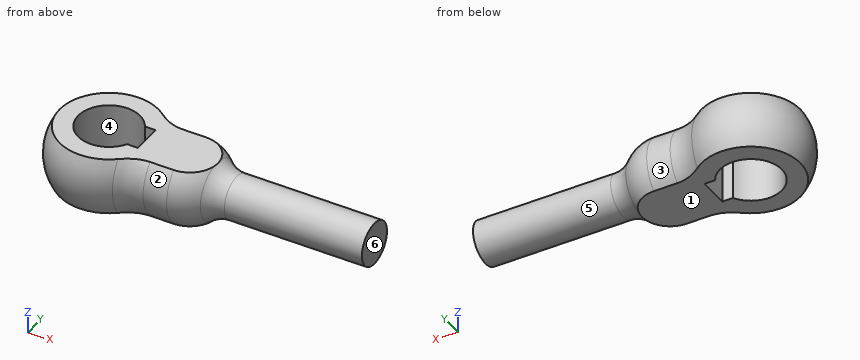
Autodesk Inventor part; units mm, degrees
ref_plane "YZ Plane" through (0, 0, 0) normal (1, 0, 0) x (0, 1, 0)
ref_plane "XZ Plane" through (0, 0, 0) normal (0, 1, 0) x (-1, 0, 0)
ref_plane "XY Plane" through (0, 0, 0) normal (0, 0, 1) x (1, 0, 0)
sketch "Эскиз1" plane through (0, 0, 0) normal (0, 0, 1) x (1, 0, 0)
  circle A0 centre (0, 0) radius 60
  circle A1 centre (0, 0) radius 32.5
  line L0 (28.2887, 16) -> (28.2887, -16)
  line L1 (28.2887, 16) -> (39.5, 16)
  line L2 (39.5, 16) -> (39.5, -16)
  line L3 (39.5, -16) -> (28.2887, -16)
  line L4 (-60, 0) -> (279.451, 0)
  line L5 (42.8486, 42) -> (42.8486, -42)
  line L6 (42.8486, 42) -> (85, 42)
  line L7 (85, 42) -> (85, -42)
  line L8 (85, -42) -> (42.8486, -42)
  line L9 (42.8486, -42) -> (42.8486, 42)
  circle A2 centre (60.2993, 92) radius 50
  line L10 (0, 0) -> (60.2993, 92)
  circle A3 centre (85, 0) radius 42
  line L11 (85, 22.5) -> (278.9533, 22.5)
  line L12 (278.9533, 22.5) -> (278.9533, -22.5)
  line L13 (278.9533, -22.5) -> (85, -22.5)
  line L14 (85, -22.5) -> (85, 22.5)
  circle A4 centre (134.2722, 52.5) radius 30
  line L15 (85, 0) -> (134.2722, 52.5)
  point P0 (-32.5, 0)
  point P1 (278.9533, 0)
  point P2 (278.9533, 0)
  point P3 (134.2722, 22.5)
  point P4 (113.7421, 30.625)
  point P5 (60.2993, 42)
  point P6 (32.8905, 50.1818)
  dimension "d17" = 84
  dimension "d0" = 120
  dimension "d1" = 65
  dimension "d2" = 32
  dimension "d3" = 72
  dimension "d4" = 84
  dimension "d7" = 100
  dimension "d8" = 92
  dimension "d10" = 110
  dimension "d11" = 85
  dimension "d12" = 0
  dimension "d13" = 45
  dimension "d14" = 60
  dimension "d15" = 52.5
  dimension "d16" = 72
  dimension "d18" = 0
revolve "Вращение1" add sketch "Эскиз1" angle 360 about axis through (-60, 0, 0) along (1, 0, 0) picked at (45.8038, 26.0598) picked at (54.3043, 5.6582) picked at (76.4143, 10.6672) picked at (29.0608, 8.9784) contours A0 L10 A1 L4 | A2 L6 A0 | A0 L5 L4 L2 L1 A1 L10 | A1 L10 L4 | L5 A0 A3 L4 | L6 A3 A0 | A1 L0 L4 L10 | L4 A3 A0 | A0 A3 L7 L4 | L4 A1 L1 L2 | A3 L15 L11 L7 | A1 L4 L0 | L15 L11 A3 L4 | L7 L11 L15 | A3 L11 L12 L4 | A4 L11 A3 | A3 L11 L15
sketch "Эскиз2" plane through (0, 0, 0) normal (0, 1, 0) x (-1, 0, 0)
  line L0 (105.3756, -30) -> (-295.1428, -30)
  line L1 (-295.1428, -30) -> (-295.1428, 30)
  line L2 (-295.1428, 30) -> (105.3756, 30)
  line L3 (105.3756, 30) -> (105.3756, -30)
  point P0 (0, 0)
  point P1 (105.3756, 0)
  point P2 (0, 0)
  dimension "d20" = 0
  dimension "d21" = 60
extrude "Выдавливание1" cut sketch "Эскиз2" along normal mid plane 200 keep common part
sketch "Эскиз3" plane through (60.2993, -29.3939, 30) normal (0, 0, 1) x (1, 0, 0)
  circle A0 centre (-60.2993, 29.3939) radius 32.5
  line L0 (-32.0106, 13.3939) -> (-32.0106, 45.3939)
  line L1 (-32.0106, 45.3939) -> (-20.7993, 45.3939)
  line L2 (-20.7993, 45.3939) -> (-20.7993, 13.3939)
  line L3 (-20.7993, 13.3939) -> (-32.0106, 13.3939)
  line L4 (-32.0106, 13.3939) -> (-32.0106, 45.3939)
  point P0 (-92.7993, 29.3939)
  point P1 (-32.0106, 13.3939)
  dimension "d24" = 65
  dimension "d25" = 32
  dimension "d26" = 72
extrude "Выдавливание2" cut sketch "Эскиз3" against normal blind 100
properties part number "1_3"
Input: part model. Units: mm. Frame: model coordinates. Face numbers are marked on the shaded views. A direction names the side the tool comes from. Coordinates: 2 decimals unless noted, no trailing zeros. Write each loop counter-clockwise with the first axis right and the second up, starting at its lowest first coordinate (ties: lowest second). Pieces come first, ordered by that corner, then holes. Notation, with made-up numbers: M -13.75,-14.75 L 30.25,-14.75 A20 ccw 30.25,1.25 Z; hole C 13.5,-3.75 d2. An arc over 180 degrees is marked long. Answer as a JSON object with one key per item and string values. Group by question number.
(1) Ray query, line 1 along Y through (x, z) = (11, -17.5); line 2 along X through (y, z) = (0.5, -17); line 3 along X through (y, z) = (-10.5, 19.5). Return the intervals inside material, ascending. Write a range as [from, to].
(2) Mould query, pull axis X, two halves, no side actions, for the marked faces 4, 5 and 6. Classes: pulls with the +X half, pulls with the -X half, needs draft (parallel to the pull), parting line crosses it, or undercut.
(3) Contact query for flat-ended pins moving along their axis: P1, Ø2, axis at x = 89.5, z = 0, coming from the -Y side; P2, Ø12, axis at x = 231.5, z = 6, coming from the -Y side; P3, Ø5.5, axis at x = 36, z = -7.5, coming from the +Y side. Output: stop coordinate, or through.
(4) Set-up query: the marked faces 1, 2 and 3. Return all of +Z, -Z, +X, -X, +Y, -Y with unobstructed straight access to the full face (end or side cutting, diameter ignored); none if empty.
(5) Section C-C on z = 0. Output: boundary loops of the cut face in (x, y) (3 decimals), plus the area to 3 significant figures.
(6) Section B-B on y = 0. Output: boundary loops of the cut face in (x, z), plus the area to 3 significant figures.
(7) Section D-D on x = 172.5. Output: boundary loops of the cut face in (y, z).
(8) Section A-A on x = 0. Output: boundary loops of the cut face in (y, z), plus the area to 3 significant figures.
Result set:
{
 "1": {"line 1": "y = [-56.33, -30.58], [30.58, 56.33]", "line 2": "x = [-57.54, -32.5], [39.5, 278.95]", "line 3": "x = [-55.76, -30.76], [39.5, 278.95]"},
 "2": {"face 4": "undercut", "face 5": "needs draft", "face 6": "pulls with the +X half"},
 "3": {"P1": "stops at y = -41.85", "P2": "stops at y = -22.5", "P3": "stops at y = 49.43"},
 "4": {"face 1": "-Z, +X, -X, +Y, -Y", "face 2": "+X, -Y", "face 3": "+X, +Y"},
 "5": {"outline": "M 32.891,-50.182 A50 cw 60.299,-42 L 85,-42 A42 ccw 113.742,-30.625 A30 cw 134.272,-22.5 L 278.953,-22.5 L 278.953,22.5 L 134.272,22.5 A30 cw 113.742,30.625 A42 ccw 85,42 L 60.299,42 A50 cw 32.891,50.182 A60 ccw long Z; hole M 28.289,-16 L 39.5,-16 L 39.5,16 L 28.289,16 A32.5 ccw long Z", "area": "20,100 mm2"},
 "6": {"outline": "M -51.96,-30 L -32.5,-30 L -32.5,30 L -51.96,30 A60 ccw Z; M 39.5,-30 L 114.43,-30 A30 cw 134.27,-22.5 L 278.95,-22.5 L 278.95,22.5 L 134.27,22.5 A30 cw 114.43,30 L 39.5,30 Z", "area": "13,500 mm2"},
 "7": {"outline": "C 0,0 d45"},
 "8": {"outline": "M -51.96,-30 L -32.5,-30 L -32.5,30 L -51.96,30 A60 ccw Z; M 32.5,-30 L 51.96,-30 A60 ccw 51.96,30 L 32.5,30 Z", "area": "2,990 mm2"}
}
